Source: CAD feature listing. Evaluate the final solid. Frame: model axes, mm. A direction names the side the tool comes from. Coordinates: 2 decimals unless noted, no trailing zeros. Order: outer loops, then holes, each group sorted by start corner. A loop starts at its lowest first (then second) coordinate and runs counter-clockwise, first axis right, second up.
```python
from build123d import *

# Parameters (mm, degrees)
F0_W     = 45
F0_H     = 18
F1_DEPTH = 4
F3_DEPTH = 2
F4_R     = 2
F5_DEPTH = 25


with BuildPart() as f1:
    # F0 (on Top) → F1 (new body)
    with BuildSketch(Plane.XY):
        Rectangle(F0_W, F0_H)
        Polygon((-12.5, 4.0414518843), (-9, 2.0207259422), (-9, -2.0207259422), (-12.5, -4.0414518843), (-16, -2.0207259422), (-16, 2.0207259422), align=None, mode=Mode.SUBTRACT)
        Polygon((12.5, 4.0414518843), (16, 2.0207259422), (16, -2.0207259422), (12.5, -4.0414518843), (9, -2.0207259422), (9, 2.0207259422), align=None, mode=Mode.SUBTRACT)
        Polygon((-9, -2.0207259422), (-9, 2.0207259422), (-12.5, 4.0414518843), (-16, 2.0207259422), (-16, -2.0207259422), (-12.5, -4.0414518843), align=None)
        Polygon((16, -2.0207259422), (16, 2.0207259422), (12.5, 4.0414518843), (9, 2.0207259422), (9, -2.0207259422), (12.5, -4.0414518843), align=None)
    extrude(amount=F1_DEPTH)

    # F2 (on face) → F3 (cut)
    with BuildSketch(Plane(origin=(0, 0, 0), x_dir=(1, 0, 0), z_dir=(0, 0, -1))):
        with BuildLine():
            ThreePointArc((-9.4689111711, -1.750000146), (-9.1192596298, -0.9058667393), (-9, 0))
            ThreePointArc((-9, 0), (-9.1192596232, 0.9058667146), (-9.4689111455, 1.7500001018))
            ThreePointArc((-9.4689111455, 1.7500001018), (-10.7500000509, 3.0310889426), (-12.5, 3.5))
            ThreePointArc((-12.5, 3.5), (-14.2499999465, 3.0310889441), (-15.5310888515, 1.750000107))
            ThreePointArc((-15.5310888515, 1.750000107), (-16, 1.113e-07), (-15.5310889628, -1.7499999142))
            ThreePointArc((-15.5310889628, -1.7499999142), (-14.2500000429, -3.0310888885), (-12.5, -3.5))
            ThreePointArc((-12.5, -3.5), (-10.750000073, -3.0310889554), (-9.4689111711, -1.750000146))
        make_face()
        with BuildLine():
            ThreePointArc((-15.5310888515, 1.750000107), (-14.2499999465, 3.0310889441), (-12.5, 3.5))
            Line((-12.5, 3.5), (-14.5207259422, 3.5))
            Line((-14.5207259422, 3.5), (-15.5310888515, 1.750000107))
        make_face()
        with BuildLine():
            ThreePointArc((-15.5310889628, -1.7499999142), (-16, 1.113e-07), (-15.5310888515, 1.750000107))
            Line((-15.5310888515, 1.750000107), (-16.5414518843, 0))
            Line((-16.5414518843, 0), (-15.5310889628, -1.7499999142))
        make_face()
        with BuildLine():
            Line((-14.5207259422, -3.5), (-12.5, -3.5))
            ThreePointArc((-12.5, -3.5), (-14.2500000429, -3.0310888885), (-15.5310889628, -1.7499999142))
            Line((-15.5310889628, -1.7499999142), (-14.5207259422, -3.5))
        make_face()
        with BuildLine():
            Line((-10.4792740578, -3.5), (-9.4689111711, -1.750000146))
            ThreePointArc((-9.4689111711, -1.750000146), (-10.750000073, -3.0310889554), (-12.5, -3.5))
            Line((-12.5, -3.5), (-10.4792740578, -3.5))
        make_face()
        with BuildLine():
            ThreePointArc((-9.4689111455, 1.7500001018), (-9.1192596232, 0.9058667146), (-9, 0))
            ThreePointArc((-9, 0), (-9.1192596298, -0.9058667393), (-9.4689111711, -1.750000146))
            Line((-9.4689111711, -1.750000146), (-8.4585481157, 0))
            Line((-8.4585481157, 0), (-9.4689111455, 1.7500001018))
        make_face()
        with BuildLine():
            ThreePointArc((-12.5, 3.5), (-10.7500000509, 3.0310889426), (-9.4689111455, 1.7500001018))
            Line((-9.4689111455, 1.7500001018), (-10.4792740578, 3.5))
            Line((-10.4792740578, 3.5), (-12.5, 3.5))
        make_face()
        with BuildLine():
            ThreePointArc((15.5310888131, -1.7500001734), (15.8807403661, -0.9058667546), (16, 0))
            ThreePointArc((16, 0), (15.8807403727, 0.9058667299), (15.5310888387, 1.7500001291))
            ThreePointArc((15.5310888387, 1.7500001291), (14.2499999354, 3.0310889505), (12.5, 3.5))
            ThreePointArc((12.5, 3.5), (10.7499999929, 3.0310889092), (9.4689110786, 1.7499999859))
            ThreePointArc((9.4689110786, 1.7499999859), (9, -1.92e-08), (9.4689110978, -1.7500000191))
            ThreePointArc((9.4689110978, -1.7500000191), (10.7500000096, -3.0310889188), (12.5, -3.5))
            ThreePointArc((12.5, -3.5), (14.2499999133, -3.0310889633), (15.5310888131, -1.7500001734))
        make_face()
        with BuildLine():
            ThreePointArc((15.5310888387, 1.7500001291), (15.8807403727, 0.9058667299), (16, 0))
            ThreePointArc((16, 0), (15.8807403661, -0.9058667546), (15.5310888131, -1.7500001734))
            Line((15.5310888131, -1.7500001734), (16.5414518843, 0))
            Line((16.5414518843, 0), (15.5310888387, 1.7500001291))
        make_face()
        with BuildLine():
            Line((14.5207259422, -3.5), (15.5310888131, -1.7500001734))
            ThreePointArc((15.5310888131, -1.7500001734), (14.2499999133, -3.0310889633), (12.5, -3.5))
            Line((12.5, -3.5), (14.5207259422, -3.5))
        make_face()
        with BuildLine():
            Line((10.4792740578, -3.5), (12.5, -3.5))
            ThreePointArc((12.5, -3.5), (10.7500000096, -3.0310889188), (9.4689110978, -1.7500000191))
            Line((9.4689110978, -1.7500000191), (10.4792740578, -3.5))
        make_face()
        with BuildLine():
            ThreePointArc((9.4689110978, -1.7500000191), (9, -1.92e-08), (9.4689110786, 1.7499999859))
            Line((9.4689110786, 1.7499999859), (8.4585481157, 0))
            Line((8.4585481157, 0), (9.4689110978, -1.7500000191))
        make_face()
        with BuildLine():
            ThreePointArc((9.4689110786, 1.7499999859), (10.7499999929, 3.0310889092), (12.5, 3.5))
            Line((12.5, 3.5), (10.4792740578, 3.5))
            Line((10.4792740578, 3.5), (9.4689110786, 1.7499999859))
        make_face()
        with BuildLine():
            ThreePointArc((12.5, 3.5), (14.2499999354, 3.0310889505), (15.5310888387, 1.7500001291))
            Line((15.5310888387, 1.7500001291), (14.5207259422, 3.5))
            Line((14.5207259422, 3.5), (12.5, 3.5))
        make_face()
    extrude(amount=-F3_DEPTH, mode=Mode.SUBTRACT)

    # F4 (on face) → F5 (cut)
    with BuildSketch(Plane(origin=(0, 0, 0), x_dir=(1, 0, 0), z_dir=(0, 0, -1))):
        with Locations((-12.5, 0)):
            Circle(F4_R)
        with Locations((12.5, 0)):
            Circle(F4_R)
    extrude(amount=-F5_DEPTH, mode=Mode.SUBTRACT)


solid = f1.part
```
Q1. Material intervals for line 1 along X through (y, z) = (0, 3.65); line 2 along Y through (x, z) = (-12.5, 3); line 3 along X through (y, z) = (-0.75, 3.7), sorted ascending.
Solutions:
line 1: x = -22.5 to -14.5, -10.5 to 10.5, 14.5 to 22.5
line 2: y = -9 to -2, 2 to 9
line 3: x = -22.5 to -14.35, -10.65 to 10.65, 14.35 to 22.5
Q2. Pull-direction query (Y, two-part tool) for faces 3 (the flat face through (-12, -3.5, 1)), 4 (the flat face through (0, 9, 2)), 5 (the flat face through (22.5, 0, 2)); classes: pulls with the +Y half, pulls with the -Y half, needs draft (parallel to the pull), parting line crosses it, or undercut.
Solutions:
face 3: undercut
face 4: pulls with the +Y half
face 5: needs draft
Q3. Section query C-C on x = 14. Output: boundary loops of the cut face in (y, z), plus the area to 3 significant figures.
Solutions:
outline: (-9, 0) - (-3.5, 0) - (-3.5, 2) - (-1.32, 2) - (-1.32, 4) - (-9, 4) - close; (1.32, 2) - (3.5, 2) - (3.5, 0) - (9, 0) - (9, 4) - (1.32, 4) - close
area: 52.7 mm2
Q4. Set-up query: faces 1 (the flat face through (-13, 3.5, 1)), 2 (the cylindrical face through (-14.1, 1.2, 3)). Return all of +Z, -Z, +X, -X, +Y, -Y with unobstructed straight access to the full face (end or side cutting, diameter ignored); none if empty.
Solutions:
face 1: -Z
face 2: +Z, -Z
Q5. Section query B-B on x = -12.5. Output: boundary loops of the cut face in (y, z).
Solutions:
outline: (-9, 0) - (-3.5, 0) - (-3.5, 2) - (-2, 2) - (-2, 4) - (-9, 4) - close; (2, 2) - (3.5, 2) - (3.5, 0) - (9, 0) - (9, 4) - (2, 4) - close
Q6. Section query A-A on z = 3.6. Output: boundary loops of the cut face in (x, y), plus the area to 3 significant figures.
Solutions:
outline: (-22.5, -9) - (22.5, -9) - (22.5, 9) - (-22.5, 9) - close; hole circle Ø4 at (-12.5, 0); hole circle Ø4 at (12.5, 0)
area: 785 mm2
Q7. Pin query (flat end, axial travel): P1, Ø3.5, axis at x = 12.5, y = 0, coming from the +Z side. Return the tip coordinate at first contact, or that it passes through.
Solutions:
P1: passes through
